Part model, mm, in its own coordinate system. Face numbers are marked on the shaded views. A direction names the side the tool comes from. Coordinates: 2 decimals unless noted, no trailing zeros. Write each loop counter-clockwise with the first axis right and the second up, starting at its lowest first coordinate (ties: lowest second). Pieces come first, ordered by that corner, then holes. Notation, with made-up numbers: (15, 57.25) - (27, 57.25) arc R20 cw to (27, 69.25) - close; hole circle Ø9 at (34.25, 15.5). An arc over 180 degrees is marked (long way). Write each question's results on one line, items separated by ' | '.
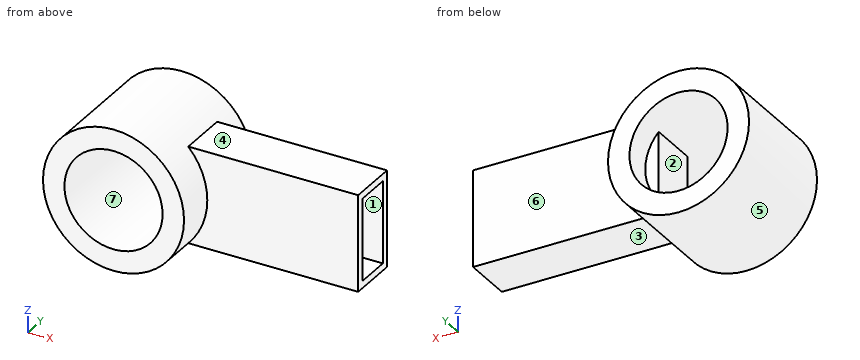
from build123d import *

# Parameters (mm, degrees)
SKETCH_356_R              = 19.75
SKETCH_356_R_2            = 13.75
EXTRUDE_6_27_5_3_10_DEPTH = 80
SKETCH_7_W                = 27
SKETCH_7_H                = 14
EXTRUDE_2_DEPTH           = 52
SKETCH_8_W                = 23
SKETCH_8_H                = 10
CUT_EXTRUDE_1_DEPTH       = 50
SKETCH_9_R                = 19.75
SKETCH_9_R_2              = 13.75
CUT_EXTRUDE_1_2_DEPTH     = 47


with BuildPart() as part:
    # Sketch 356 → 6分管 內直徑27.5厚度3長度10 (new body)
    with BuildSketch(Plane(origin=(0, 0, 0), x_dir=(1, 0, 0), z_dir=(0, 1, 0))):
        Circle(SKETCH_356_R)
        Circle(SKETCH_356_R_2, mode=Mode.SUBTRACT)
    extrude(amount=EXTRUDE_6_27_5_3_10_DEPTH)

    # 草圖7 → 填料-伸長2 (add)
    with BuildSketch(Plane(origin=(10, 0, 0), x_dir=(0, 0, -1), z_dir=(1, 0, 0))):
        with Locations((0, 65.299252319)):
            Rectangle(SKETCH_7_W, SKETCH_7_H)
    extrude(amount=EXTRUDE_2_DEPTH)

    # 草圖8 → Cut-Extrude 1 (cut)
    with BuildSketch(Plane(origin=(62, 0, 0), x_dir=(0, 0, -1), z_dir=(1, 0, 0))):
        with Locations((0, 65.299252319)):
            Rectangle(SKETCH_8_W, SKETCH_8_H)
    extrude(amount=-CUT_EXTRUDE_1_DEPTH, mode=Mode.SUBTRACT)

    # 草圖9 → Cut-Extrude 1 2 (cut)
    with BuildSketch(Plane.XZ):
        Circle(SKETCH_9_R)
        Circle(SKETCH_9_R_2, mode=Mode.SUBTRACT)
    extrude(amount=-CUT_EXTRUDE_1_2_DEPTH, mode=Mode.SUBTRACT)


solid = part.part
(1) Saw through at B-B on z = 0. Write the cut outline in (x, y).
Return value:
outline: (-19.75, 47) - (-13.75, 47) - (-13.75, 80) - (-19.75, 80) - close; (10, 58.3) - (13.75, 58.3) - (13.75, 47) - (19.75, 47) - (19.75, 58.3) - (62, 58.3) - (62, 60.3) - (12, 60.3) - (12, 70.3) - (62, 70.3) - (62, 72.3) - (19.75, 72.3) - (19.75, 80) - (13.75, 80) - (13.75, 72.3) - (10, 72.3) - close
(2) Wall check: line 1 (Z direction, x = 0, y = 58); line 2 (X direction, y = 52.5, z = -0.5); line 3 (X direction, y = 65.5, z = 0). Give the ranges that are in metal, low to high. Write a range as from..to.
Return value:
line 1: z = -19.75..-13.75, 13.75..19.75 | line 2: x = -19.74..-13.74, 13.74..19.74 | line 3: x = -19.75..-13.75, 10..12
(3) Two-plate mould, pull along X, no slides. Class the marked faces 5, 6 and 7: released by +X, released by -X, zero draft, split by the parting line, or undercut.
Return value:
face 5: split by the parting line | face 6: zero draft | face 7: undercut
(4) Flat gauge pins, fed straight in: P1, Ø6, axis at y = 76, z = 12.5, coming from the -X side; P2, Ø11, axis at x = 48.5, y = 63, coming from the -Z side; P3, Ø5, axis at y = 66.5, z = 3.5, coming from the +X side; P4, Ø1.5, axis at x = 22, z = 15, coming from the +Y side. Where does each tip first touch, or does it go through?
Return value:
P1: stops at x = -17.32 | P2: stops at z = -13.5 | P3: stops at x = 12 | P4: passes through
(5) Saw through at D-D on z = -15.5. Write the cut outline in (x, y), then the cut area to 3 significant figures.
Return value:
outline: (-12.24, 47) - (12.24, 47) - (12.24, 80) - (-12.24, 80) - close | area: 808 mm^2
(6) Saw through at A-A on y = 62.5. Write the cut outline in (x, z).
Return value:
outline: (12, -11.5) - (12, 11.5) - (62, 11.5) - (62, 13.5) - (14.42, 13.5) arc R19.75 ccw (long way) to (14.42, -13.5) - (62, -13.5) - (62, -11.5) - close; hole (10, -9.44) - (10, 9.44) arc R13.75 ccw (long way) to start
(7) 3-axis set-ups, long thin cutter, end or side, ignore diameter. For the marked faces 1, 2, 3 and 4: which of +Z, -Z, +X, -X, +Y, -Y reach the whole face in a straight line?
Return value:
face 1: +X | face 2: +Y, -Y | face 3: -Z, +X, +Y, -Y | face 4: +Z, +X, +Y, -Y
(8) Saw through at C-C on x = 0. Write the cut outline in (y, z), then the cut area to 3 significant figures.
Return value:
outline: (47, -19.75) - (80, -19.75) - (80, -13.75) - (47, -13.75) - close; (47, 13.75) - (80, 13.75) - (80, 19.75) - (47, 19.75) - close | area: 396 mm^2
